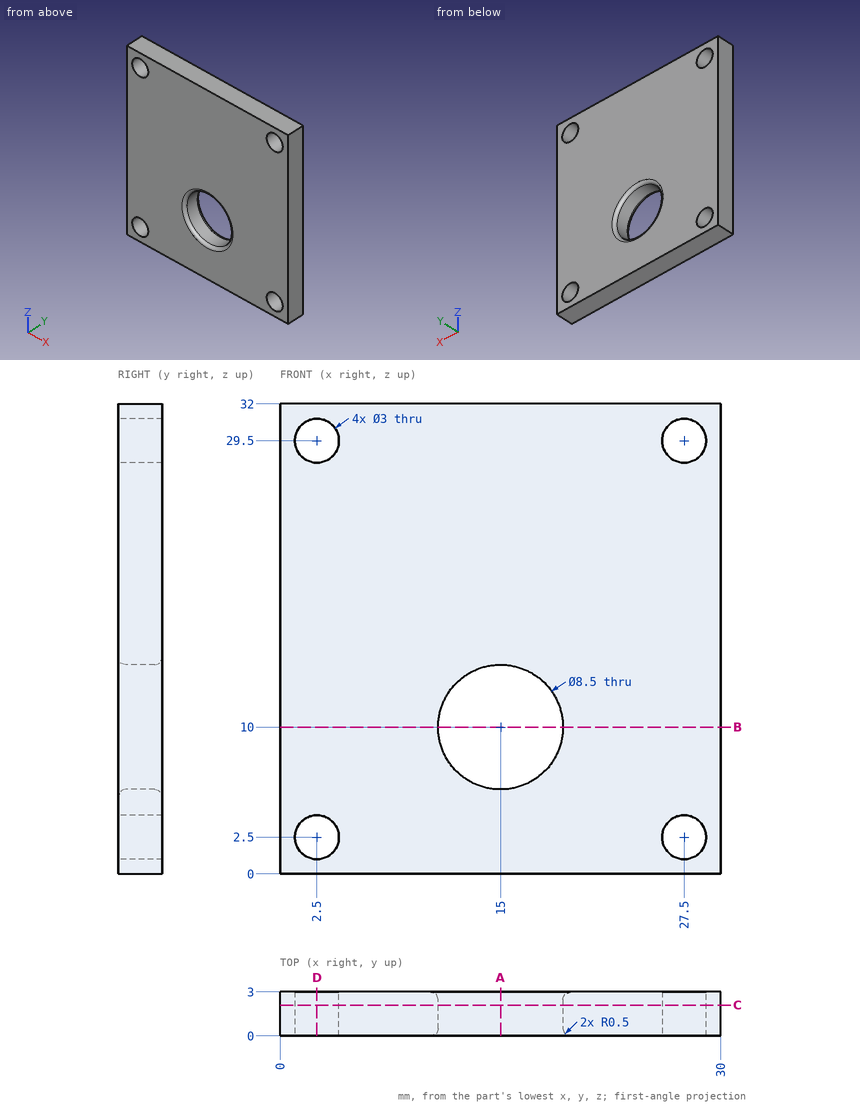
Job drawing, mm, ordinate dimensions from the low corner. One solid piece. Round coordinates to 2 decimals unless told otherwise and drop trailing zeros. Write each loop counter-clockwise with the first axis right and the second up, starting at its lowest first coordinate (ties: lowest second). Pieces come first, ordered by that corner, then holes.
1) Band-saw the part on A-A, the plane x = 15. List the corners of the cut face in (y, z), and give its area (3 significant figures).
2) Band-saw the part on D-D, the plane x = 2.5. List the corners of the cut face in (y, z).
3) Pin check, flat tip, straight feed: pin 1 (2.5 mm diameter, centred on x = 27.5, z = 29.5, fed in from -Y). Stop position of the tip, or through.
4) Band-saw the part on C-C, the plane y = 2.1. List the corners of the cut face in (x, z).
5) Band-saw the part on B-B, the plane z = 10. List the corners of the cut face in (x, y), and give its area (3 significant figures).
6) Drill centre lines: probe 1 along X at (y, z) = (2.15, 2.5); probe 2 along Z at (x, y) = (2.5, 2.35); probe 3 along X at (y, z) = (0.8, 29). Where is each one in solid material? Low to high.
Ans:
1. outline: (0, 0) - (3, 0) - (3, 5.25) arc R0.5 ccw to (2.5, 5.75) - (0.5, 5.75) arc R0.5 ccw to (0, 5.25) - close; (0, 14.75) arc R0.5 ccw to (0.5, 14.25) - (2.5, 14.25) arc R0.5 ccw to (3, 14.75) - (3, 32) - (0, 32) - close
1. area: 70.3 mm2
2. outline: (0, 0) - (3, 0) - (3, 1) - (0, 1) - close; (0, 4) - (3, 4) - (3, 28) - (0, 28) - close; (0, 31) - (3, 31) - (3, 32) - (0, 32) - close
3. pin 1: passes through
4. outline: (0, 0) - (30, 0) - (30, 32) - (0, 32) - close; hole circle Ø3 at (2.5, 2.5); hole circle Ø3 at (2.5, 29.5); hole circle Ø8.5 at (15, 10); hole circle Ø3 at (27.5, 2.5); hole circle Ø3 at (27.5, 29.5)
5. outline: (0, 0) - (10.25, 0) arc R0.5 ccw to (10.75, 0.5) - (10.75, 2.5) arc R0.5 ccw to (10.25, 3) - (0, 3) - close; (19.25, 0.5) arc R0.5 ccw to (19.75, 0) - (30, 0) - (30, 3) - (19.75, 3) arc R0.5 ccw to (19.25, 2.5) - close
5. area: 64.3 mm2
6. probe 1: x = 0 to 1, 4 to 26, 29 to 30
6. probe 2: z = 0 to 1, 4 to 28, 31 to 32
6. probe 3: x = 0 to 1.09, 3.91 to 26.09, 28.91 to 30
